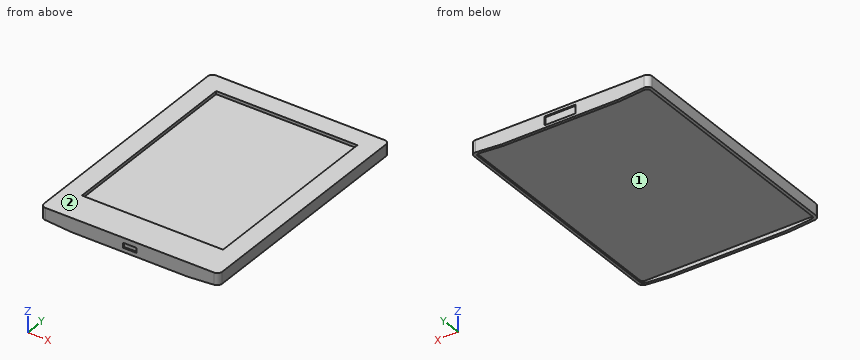
```python
from build123d import *

# Parameters (mm, degrees)
PAD_DEPTH       = 78.2
PAD_DEPTH_BACK  = 78.2
SKETCH004_W     = 91
SKETCH004_H     = 123.3
POCKET_DEPTH    = 2
POCKET001_DEPTH = 2.6
FILLET_R        = 3
SKETCH012_W     = 8.6
SKETCH012_H     = 3.2
POCKET003_DEPTH = 1
SKETCH013_W     = 20
SKETCH013_H     = 5.6
POCKET004_DEPTH = 1


with BuildPart() as part:
    # Sketch003 → Pad (new body, two sides)
    with BuildSketch(Plane.XZ) as pad_sk:
        Polygon((-57.4, 6.4), (57.4, 6.4), (57.4, -1.1), (37.4, -2.6), (-37.4, -2.6), (-57.4, -1.1), align=None)
    extrude(amount=PAD_DEPTH)
    extrude(pad_sk.sketch, amount=-PAD_DEPTH_BACK)

    # Sketch004 (on Face2 of Pad) → Pocket (cut)
    with BuildSketch(Plane(origin=(0, 0, 6.4), x_dir=(-1, 0, 0), z_dir=(0, 0, 1))):
        with Locations((0, -4.25)):
            Rectangle(SKETCH004_W, SKETCH004_H)
    extrude(amount=-POCKET_DEPTH, mode=Mode.SUBTRACT)

    # Sketch005 (on Face6 of Pocket) → Pocket001 (cut)
    with BuildSketch(Plane(origin=(0, 0, -2.6), x_dir=(1, 0, 0), z_dir=(0, 0, -1))):
        with BuildLine():
            Line((-53.5, 76.4), (53.5, 76.4))
            ThreePointArc((55.5, 74.4), (54.914214, 75.814214), (53.5, 76.4))
            Line((55.5, 74.4), (55.5, -74.4))
            ThreePointArc((53.5, -76.4), (54.914214, -75.814214), (55.5, -74.4))
            Line((53.5, -76.4), (-53.5, -76.4))
            ThreePointArc((-55.5, -74.4), (-54.914214, -75.814214), (-53.5, -76.4))
            Line((-55.5, -74.4), (-55.5, 74.4))
            ThreePointArc((-53.5, 76.4), (-54.914214, 75.814214), (-55.5, 74.4))
        make_face()
    extrude(amount=-POCKET001_DEPTH, mode=Mode.SUBTRACT)

    # Fillet
    fillet_edges = [part.edges().sort_by_distance(p)[0] for p in [
        (57.4, -78.2, 2.65),
        (57.4, 78.2, 2.65),
        (-57.4, -78.2, 2.65),
        (-57.4, 78.2, 2.65),
    ]]
    fillet(fillet_edges, radius=FILLET_R)

    # Sketch012 (on Face10 of Fillet) → Pocket003 (cut)
    with BuildSketch(Plane.XZ.offset(78.2)):
        with Locations((0, 1.6)):
            Rectangle(SKETCH012_W, SKETCH012_H)
    extrude(amount=-POCKET003_DEPTH, mode=Mode.SUBTRACT)

    # Sketch013 (on Face6 of Pocket003) → Pocket004 (cut)
    with BuildSketch(Plane(origin=(0, 78.2, 0), x_dir=(1, 0, 0), z_dir=(0, 1, 0))):
        with Locations((0, -1.8)):
            Rectangle(SKETCH013_W, SKETCH013_H)
    extrude(amount=-POCKET004_DEPTH, mode=Mode.SUBTRACT)


with BuildPart() as part_1:
    # Body003 placement: moved
    add(part.part.moved(Location((0, 0, 12))))


solid = part_1.part
```
For this review, take the finished solid that the model builds, in its own axes (mm). Face numbers are marked on the shaded views. Round coordinates to 2 decimals unless told otherwise and drop trailing zeros. Write each loop counter-clockwise with the first axis right and the second up, starting at its lowest first coordinate (ties: lowest second). Pieces come first, ordered by that corner, then holes. Notation, with made-up numbers: (-20.75, 25) -> (3.25, 25) arc R34 cw to (3.25, 64) -> close; hole circle Ø10 at (85.5, 26.25). An arc over 180 degrees is marked (long way). One line per question, with ' | ' between items. Start each with the question number.
(1) Add section A-A, the plane y = 33. Write out the cut boundary in (x, z).
(2) Mouldability with a two-part tool opening along Y and no side actions: class the marked faces 1 and 2 as released by +Y, released by -Y, zero draft, split by the parting line, or undercut.
(3) For line 1 along Y through (x, z) = (-40, 16.75); line 2 along Y through (x, z) = (-1, 11.5); line 3 along Z through (x, y) = (-42.5, 46), list the stretches that pass through material, from the lowest coordinate up. Write a range as from..to.
(4) Insertion check: P1, Ø1.7, axis at x = -4, z = 13, coming from the +Y side; P2, Ø1.1, axis at y = -77.5, z = 13.5, coming from the +X side; P3, Ø3, axis at x = -26, y = 14, coming from the -Z side. Each pin has a flat end and moves straight along its axis. Give the tip position at first contact, or say it passes through.
(5) Add section B-B, the plane x = 27. Write out the cut boundary in (y, z), plus the area to 3 significant figures.
Answer list:
1) outline: (-57.4, 10.9) -> (-55.5, 10.76) -> (-55.5, 12) -> (55.5, 12) -> (55.5, 10.76) -> (57.4, 10.9) -> (57.4, 18.4) -> (45.5, 18.4) -> (45.5, 16.4) -> (-45.5, 16.4) -> (-45.5, 18.4) -> (-57.4, 18.4) -> close
2) face 1: undercut | face 2: zero draft
3) line 1: -78.2..-57.4, 65.9..78.2 | line 2: -78.2..-76.4, 76.4..77.2 | line 3: 12..16.4
4) P1: y = 77.2 | P2: x = 56.84 | P3: z = 12
5) outline: (-78.2, 9.4) -> (-76.4, 9.4) -> (-76.4, 12) -> (76.4, 12) -> (76.4, 9.4) -> (78.2, 9.4) -> (78.2, 18.4) -> (65.9, 18.4) -> (65.9, 16.4) -> (-57.4, 16.4) -> (-57.4, 18.4) -> (-78.2, 18.4) -> close | area: 764 mm²
